```python
from build123d import *

# Parameters (mm, degrees)
F0_W      = 150
F0_H      = 260
F1_DEPTH  = 18.5
F2_R      = 10
F3_DEPTH  = 25.4
F4_R      = 24.75
F5_DEPTH  = 25.4
F6_R      = 37.5
F7_DEPTH  = 11.5
F8_R      = 3.5
F9_DEPTH  = 25.4
F10_R     = 4.75
F10_R_2   = 3.5
F11_DEPTH = 6


with BuildPart() as f1:
    # F0 (on Top) → F1 (new body)
    with BuildSketch(Plane.XY):
        with Locations((75, 130)):
            Rectangle(F0_W, F0_H)
    extrude(amount=F1_DEPTH)

    # F2 (on face) → F3 (cut)
    with BuildSketch(Plane.XY.offset(18.5)):
        with Locations((75, 240)):
            Circle(F2_R)
        with Locations((75, 20)):
            Circle(F2_R)
    extrude(amount=-F3_DEPTH, mode=Mode.SUBTRACT)

    # F4 (on face) → F5 (cut)
    with BuildSketch(Plane.XY.offset(18.5)):
        with Locations((75, 172)):
            Circle(F4_R)
        with Locations((75, 88)):
            Circle(F4_R)
    extrude(amount=-F5_DEPTH, mode=Mode.SUBTRACT)

    # F6 (on face) → F7 (cut)
    with BuildSketch(Plane(origin=(0, 0, 0), x_dir=(1, 0, 0), z_dir=(0, 0, -1))):
        with Locations((75, -88)):
            Circle(F6_R)
        with Locations((75, -172)):
            Circle(F6_R)
    extrude(amount=-F7_DEPTH, mode=Mode.SUBTRACT)

    # F8 (on face) → F9 (cut)
    with BuildSketch(Plane(origin=(0, 0, 11.5), x_dir=(1, 0, 0), z_dir=(0, 0, -1))):
        with Locations((106.125, -88)):
            Circle(F8_R)
        with Locations((59.4375, -61.0449593072)):
            Circle(F8_R)
        with Locations((59.4375, -114.9550406928)):
            Circle(F8_R)
    extrude(amount=-F9_DEPTH, mode=Mode.SUBTRACT)

    # F10 (on face) → F11 (cut)
    with BuildSketch(Plane.XY.offset(18.5)):
        with Locations((59.4375, 61.0449593072)):
            Circle(F10_R)
        with Locations((59.4375, 61.0449593072)):
            Circle(F10_R_2, mode=Mode.SUBTRACT)
        with Locations((59.4375, 114.9550406928)):
            Circle(F10_R)
        with Locations((59.4375, 114.9550406928)):
            Circle(F10_R_2, mode=Mode.SUBTRACT)
        with Locations((106.125, 88)):
            Circle(F10_R)
        with Locations((106.125, 88)):
            Circle(F10_R_2, mode=Mode.SUBTRACT)
    extrude(amount=-F11_DEPTH, mode=Mode.SUBTRACT)


solid = f1.part
```
Model file for the job. Use its own axes, mm. A direction names the side the tool comes from. Give positions to 0.01 mm unless a question says otherwise; leave off trailing zeros. Write each loop counter-clockwise with the first axis right and the second up, starting at its lowest first coordinate (ties: lowest second). Pieces come first, ordered by that corner, then holes. Notation, with made-up numbers: (-2.5, 64) - (38.5, 64) arc R32 cw to (38.5, 92) - close; hole circle Ø9 at (12, 26.5). An arc over 180 degrees is marked (long way). One line per question, with ' | ' between items. Start each with the question number.
(1) Slice it at A-A on y = 172. Write the cut outline in (x, z).
(2) Slice it at B-B on x = 75. Write the cut outline in (y, z).
(3) Wall check: line 1 along Y through (x, z) = (75, 15); line 2 along Y through (x, z) = (107, 8.75); line 3 along Y through (x, z) = (42.5, 3.75). Give the ranges that are in metal, low to high. Write a range as from..to.
(4) Two-plate mould, pull along Y, no slides. Class faces 1 (the face through (74, 132, 18.5)), 2 (the face through (95.16, 140.38, 5.67)), 3 (the face through (71.78, 196.54, 15.05)), 4 (the face through (74, 0, 9)): +Y half, -Y half, draft (parallel to the pull), parting line (faces both ways), or undercut.
(5) 3-axis set-ups, long thin cutter, end or side, ignore diameter. For faces 5 (the face through (58.819, 119.665, 15.542)), 6 (the face through (83, 112, 11.5)), 7 (the face through (65, 240, 9)): which of +Z, -Z, +X, -X, +Y, -Y reach the whole face in a straight line?
(6) Slice it at C-C on z = 5. Write the cut outline in (x, y), plus the area to 3 significant figures.
(7) Slice it at D-D on y = 88. Write the cut outline in (x, z) (3 decimals), plus the area to 3 significant figures.
Results below:
1) outline: (0, 0) - (37.5, 0) - (37.5, 11.5) - (50.25, 11.5) - (50.25, 18.5) - (0, 18.5) - close; (99.75, 11.5) - (112.5, 11.5) - (112.5, 0) - (150, 0) - (150, 18.5) - (99.75, 18.5) - close
2) outline: (0, 0) - (10, 0) - (10, 18.5) - (0, 18.5) - close; (30, 0) - (50.5, 0) - (50.5, 11.5) - (63.25, 11.5) - (63.25, 18.5) - (30, 18.5) - close; (112.75, 11.5) - (125.5, 11.5) - (125.5, 0) - (134.5, 0) - (134.5, 11.5) - (147.25, 11.5) - (147.25, 18.5) - (112.75, 18.5) - close; (196.75, 11.5) - (209.5, 11.5) - (209.5, 0) - (230, 0) - (230, 18.5) - (196.75, 18.5) - close; (250, 0) - (260, 0) - (260, 18.5) - (250, 18.5) - close
3) line 1: 0..10, 30..63.25, 112.75..147.25, 196.75..230, 250..260 | line 2: 0..68.45, 107.55..152.45, 191.55..260 | line 3: 0..69.29, 106.71..153.29, 190.71..260
4) face 1: draft | face 2: undercut | face 3: undercut | face 4: -Y half
5) face 5: +Z | face 6: -Z | face 7: +Z, -Z
6) outline: (0, 0) - (150, 0) - (150, 260) - (0, 260) - close; hole circle Ø75 at (75, 88); hole circle Ø75 at (75, 172); hole circle Ø20 at (75, 20); hole circle Ø20 at (75, 240) | area: 29,500 mm^2
7) outline: (0, 0) - (37.5, 0) - (37.5, 11.5) - (50.25, 11.5) - (50.25, 18.5) - (0, 18.5) - close; (99.75, 11.5) - (102.625, 11.5) - (102.625, 12.5) - (101.375, 12.5) - (101.375, 18.5) - (99.75, 18.5) - close; (109.625, 11.5) - (112.5, 11.5) - (112.5, 0) - (150, 0) - (150, 18.5) - (110.875, 18.5) - (110.875, 12.5) - (109.625, 12.5) - close | area: 1,500 mm^2
